Can you work these out from the drawing? Everything is in mm from the part's minimum corner. A direction names the side the tool comes from. Give positions to 0.01 mm unless a question says otherwise; leave off trailing zeros. Order: outer loops, then holes, each group sorted by start corner. A loop starts at its lowest first (then second) coordinate and runs counter-clockwise, first axis right, second up. Notation, with made-up numbers: (16.5, 62) - (61.5, 62) arc R30 cw to (61.5, 86) - close; hole circle Ø1 at (30.5, 42). An arc over 180 degrees is marked (long way). Answer as a JSON object with one key per item and string values.
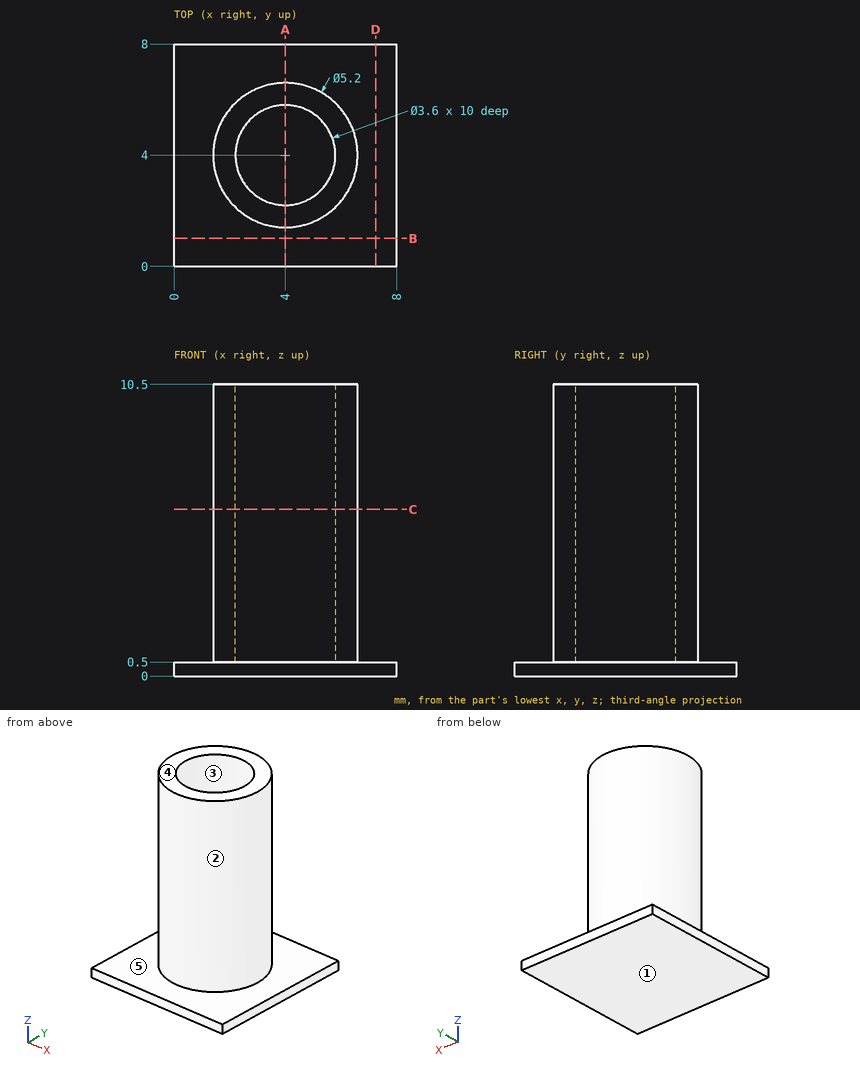
Q1. If we section it at A-A, the plane x = 4: Please give me the cut outline in (y, z), then the cut area to 3 significant figures.
Recorded:
{"outline": "(0, 0) - (8, 0) - (8, 0.5) - (6.6, 0.5) - (6.6, 10.5) - (5.8, 10.5) - (5.8, 0.5) - (2.2, 0.5) - (2.2, 10.5) - (1.4, 10.5) - (1.4, 0.5) - (0, 0.5) - close", "area": "20.0 mm^2"}
Q2. If we section it at C-C, the plane z = 6: Please give me the cut outline in (x, y), then the cut area to 3 significant figures.
Recorded:
{"outline": "circle Ø5.2 at (4, 4); hole circle Ø3.6 at (4, 4)", "area": "11.1 mm^2"}
Q3. Which directions (+Z, -Z, +X, -X, +Y, -Y) give clear straight access to the entire face, cutting with the end or side of a thin tool? Please do the marked faces 4 and 5.
Recorded:
{"face 4": "+Z, +X, -X, +Y, -Y", "face 5": "+Z"}
Q4. If we section it at B-B, the plane y = 1: Please give me the cut outline in (x, z).
Recorded:
{"outline": "(0, 0) - (8, 0) - (8, 0.5) - (0, 0.5) - close"}
Q5. I'm going to push a flat-ended pin straight in: pin 1 Ø4 at (y, z) = (4, 5.5) entering from +X. Where does the tip first touch, or does it pass through?
Recorded:
{"pin 1": "stops at x = 6.6"}
Q6. I need wall thicknesses on L1, parallel to Y at x = 4, z = 6.25; L2, parallel to Z at x = 5.25, y = 4.5; L3, parallel to X at y = 3, z = 1.25. Which ranges of each line are inside material? Lowest first, please.
Recorded:
{"L1": "y = 1.4 to 2.2, 5.8 to 6.6", "L2": "z = 0 to 0.5", "L3": "x = 1.6 to 2.5, 5.5 to 6.4"}
Q7. We'd pull the mould along X, two halves only. Please class the marked faces 1, 2 and 3: released by +X, released by -X, zero draft, split by the parting line, or undercut.
Recorded:
{"face 1": "zero draft", "face 2": "split by the parting line", "face 3": "undercut"}
